CAD build for the part. Positions are in the model's coordinates, mm. Give positions to 0.01 mm unless a question says otherwise; leave off trailing zeros. Loops run counter-clockwise (first coordinate to the right, second up) from the corner with the lowest first, then second, coordinate; pieces in that order, holes last. Notation, with made-up numbers: (-40, 62) - (4, 62) arc R34 ccw to (4, 97) - close; hole circle Ø11 at (74.5, -38.75). An arc over 180 degrees is marked (long way). Return JSON: item names as keys, results as strings.
from build123d import *

# Parameters (mm, degrees)
F0_W       = 139.7
F0_H       = 86.36
F1_DEPTH   = 228.6
F2_SIZE2   = 69.72299
F2_SIZE    = 228.59999
F2_2_SIZE2 = 69.72299
F2_2_SIZE  = 228.59999
F3_SIZE2   = 228.59999
F3_SIZE    = 43.17999


# Not quite as in the source:
# - a fillet or chamfer is up to 0.001 mm smaller than in the source, because OpenCascade refuses the exact size


with BuildPart() as f1:
    # F0 (on Top) → F1 (new body)
    with BuildSketch(Plane.XY):
        Rectangle(F0_W, F0_H)
    extrude(amount=F1_DEPTH)

    # F2 (size 228.6 and 69.723 in the source; OpenCascade refuses exactly that, so slightly less here)
    f2_edges = [f1.edges().sort_by_distance(p)[0] for p in [
        (69.85, 0, 228.6),
    ]]
    f2_side = f1.faces().sort_by_distance((69.85, 0, 114.3))[0]
    chamfer(f2_edges, length=F2_SIZE, length2=F2_SIZE2, reference=f2_side)

    # F2#2 (size 228.6 and 69.723 in the source; OpenCascade refuses exactly that, so slightly less here)
    f2_2_edges = [f1.edges().sort_by_distance(p)[0] for p in [
        (-69.85, 0, 228.6),
    ]]
    f2_2_side = f1.faces().sort_by_distance((-69.85, 0, 114.3))[0]
    chamfer(f2_2_edges, length=F2_2_SIZE, length2=F2_2_SIZE2, reference=f2_2_side)

    # F3 (size 43.18 and 228.6 in the source; OpenCascade refuses exactly that, so slightly less here)
    f3_edges = [f1.edges().sort_by_distance(p)[0] for p in [
        (0, -43.18, 228.6),
        (0, 43.18, 228.6),
    ]]
    f3_side = f1.faces().sort_by_distance((0, 0, 228.6))[0]
    chamfer(f3_edges, length=F3_SIZE, length2=F3_SIZE2, reference=f3_side)


solid = f1.part
1. Cut at D-D, the plane z = 45.5. Write the cut outline in (x, y).
Values follow:
{"outline": "(-55.97, -34.59) - (55.97, -34.59) - (55.97, 34.59) - (-55.97, 34.59) - close"}
2. Drop flat-ended pins along their axis: P1, Ø2, axis at x = 21, z = 127.5, coming from the -Y side; P2, Ø6, axis at y = 23.5, z = 86, coming from the -X side (3 decimals); P3, Ø4, axis at x = 28, z = 57, coming from the +Y side. Give the stop position or say it passes through.
Values follow:
{"P1": "stops at y = -19.29", "P2": "stops at x = -44.535", "P3": "stops at y = 32.79"}
3. Cut at C-C, the plane z = 18. Write the cut outline in (x, y).
Values follow:
{"outline": "(-64.36, -39.78) - (64.36, -39.78) - (64.36, 39.78) - (-64.36, 39.78) - close"}
4. Drill centre lines: probe 1 along Y at (x, z) = (-22, 73.5); probe 2 along X at (y, z) = (15.5, 74); probe 3 along X at (y, z) = (3, 83.5). Where is each one in solid material? Low to high.
Values follow:
{"probe 1": "y = -29.3 to 29.3", "probe 2": "x = -47.28 to 47.28", "probe 3": "x = -44.38 to 44.38"}
